Geometry check sheet. Reference: the model listing, model coordinates, mm. Round coordinates to 2 decimals unless told otherwise and drop trailing zeros. Order: outer loops, then holes, each group sorted by start corner. A loop starts at its lowest first (then second) coordinate and runs counter-clockwise, first axis right, second up. Notation, with made-up numbers: (3, 89.25) - (52, 89.25) arc R22 ccw to (52, 127.25) - close; hole circle Ø10 at (45.25, -32). An arc over 180 degrees is marked (long way). Use a Markdown table: item, result. Add a question column.
(1) Section check A-A on x = 0. Record the boundary of the cut face in (y, z).
(2) Thickness scan on line 1 along Y through (x, z) = (0, 13.5); line 2 along Z through (x, y) = (-1, -20). Record the ranges inside material, lowest first. Write a range as [from, to].
(3) Mould release check, pull along Y, two halves, no side actions. Record for faces 1 (the face through (0.568, -25.091, 28.806)), 2 (the face through (5, -50, 2)), 3 (the face through (5, -25, -27.769)), 4 (the face through (0.542, -24.972, 0.062)): released by +Y, released by -Y, zero draft, split by the parting line, or undercut.
```python
from build123d import *

# Parameters (mm, degrees)
F0_W           = 67.286568
F0_H           = 58.953825
F1_DEPTH       = 50
F3_D           = 5
F3_CSINK_D     = 10
F3_CSINK_ANGLE = 90


with BuildPart() as f1:
    # F0 (on Front) → F1 (new body)
    with BuildSketch(Plane.XZ):
        with Locations((5.915298, 1.707598)):
            Rectangle(F0_W, F0_H)
    extrude(amount=F1_DEPTH)

    # F3 (through all)
    with Locations(Plane.XY.offset(31.184511)):
        with Locations((0, -22.531725)):
            CounterSinkHole(F3_D / 2, F3_CSINK_D / 2, counter_sink_angle=F3_CSINK_ANGLE)


solid = f1.part
```
Check sheet entries:
| question | item | result |
|---|---|---|
| 1 | outline | (-50, -27.77) - (-25.03, -27.77) - (-25.03, 28.68) - (-27.53, 31.18) - (-50, 31.18) - close; (-20.03, -27.77) - (0, -27.77) - (0, 31.18) - (-17.53, 31.18) - (-20.03, 28.68) - close |
| 2 | line 1 | y = [-50, -25.03], [-20.03, 0] |
| 2 | line 2 | z = [-27.77, 28.91] |
| 3 | face 1 | undercut |
| 3 | face 2 | released by -Y |
| 3 | face 3 | zero draft |
| 3 | face 4 | undercut |
